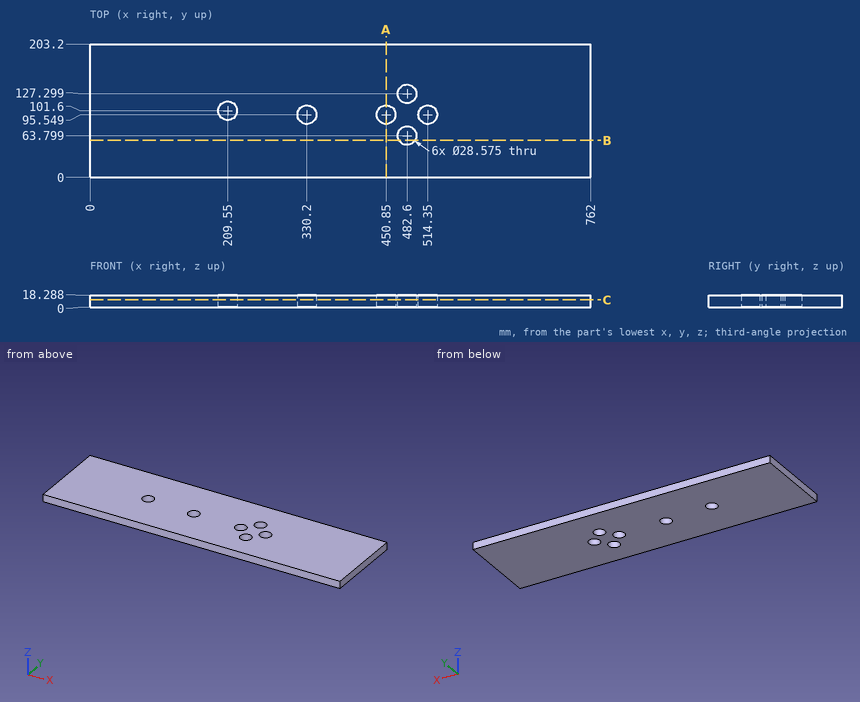
Input: dimensioned drawing with shaded views. Units: mm. Origin: part minimum x, y, z. Coordinates: 2 decimals unless noted, no trailing zeros. Write each loop counter-clockwise with the first axis right and the second up, starting at its lowest first coordinate (ties: lowest second). Pieces come first, ordered by that corner, then holes. Notation, with made-up numbers: M 21.5,10.5 L 74.5,10.5 A16 ccw 74.5,23.5 Z; hole C -11,64 d11. An arc over 180 degrees is marked long. Use a Markdown table: item, result.
1) Section B-B, the plane y = 56.5. Output: boundary loops of the cut face in (x, z).
Conclusion:
| item | result |
|---|---|
| outline | M 0,0 L 470.32,0 L 470.32,18.29 L 0,18.29 Z; M 494.88,0 L 762,0 L 762,18.29 L 494.88,18.29 Z |
2) Section C-C, the plane z = 11.5. Give the number of separate pieces and of enclosed holes in the cut face, then the cut area to 3 significant figures.
Conclusion:
| item | result |
|---|---|
| separate pieces | 1 |
| enclosed holes | 6 |
| area | 151,000 mm^2 |
3) Section A-A, the plane x = 450.85. Output: boundary loops of the cut face in (y, z).
Conclusion:
| item | result |
|---|---|
| outline | M 0,0 L 81.26,0 L 81.26,18.29 L 0,18.29 Z; M 109.84,0 L 203.2,0 L 203.2,18.29 L 109.84,18.29 Z |
4) Ray query, L1, parallel to Y at x = 482.6, z = 5; L2, parallel to Y at x = 209.55, z = 4; L3, parallel to Y at x = 451, z = 16.75. Return the intervals inside material, ascending.
Conclusion:
| item | result |
|---|---|
| L1 | y = 0 to 49.51, 78.09 to 113.01, 141.59 to 203.2 |
| L2 | y = 0 to 87.31, 115.89 to 203.2 |
| L3 | y = 0 to 81.26, 109.84 to 203.2 |
